```python
from build123d import *

# Parameters (mm, degrees)
CYLINDER014_R     = 1.5
CYLINDER014_DEPTH = 10


with BuildPart() as zylinder014:
    # Cylinder014 → Cylinder014 (new body)
    with BuildSketch(Plane.XY.offset(-17)):
        Circle(CYLINDER014_R)
    extrude(amount=CYLINDER014_DEPTH)


with BuildPart() as cut016:
    # Sketch006 → Revolve001 (revolve)
    with BuildSketch(Plane.XZ):
        Polygon((0, 0), (-3.81, 0), (-5.029301, -1.843205), (-3.199301, -1.843205), (-2.41, -6.74), (-2.41, -14.07), (0, -14.07), align=None)
    revolve(axis=Axis((0, 0, 0), (0, 0, 1)))

    # Cut016: cut Zylinder014
    add(zylinder014.part, mode=Mode.SUBTRACT)


with BuildPart() as cut016_1:
    # Cut016 placement: moved
    add(cut016.part.moved(Location((0, 0, 27.5))))


solid = cut016_1.part
```
The listing builds one solid part. Answer for the finished solid, in the listing's coordinates (mm). A direction names the side the tool comes from. Coordinates: 2 decimals unless noted, no trailing zeros. Write each loop counter-clockwise with the first axis right and the second up, starting at its lowest first coordinate (ties: lowest second). Pieces come first, ordered by that corner, then holes.
Q1. Which of the six approach directions +Z, -Z, +X, -X, +Y, -Y give full straight-line access (tool end or side, diameter ignored) to faces 1 (the flat face through (0, 2, 13.43)), 2 (the flat face through (-1, 3.3, 25.657))?
Returned:
face 1: -Z, +X, -X, +Y, -Y
face 2: -Z
Q2. Section A-A, the plane y = 0 is taken. Write down the section's boundary in (x, z), then the cut area to 3 significant figures.
Returned:
outline: (-5.03, 25.66) - (-3.2, 25.66) - (-2.41, 20.76) - (-2.41, 13.43) - (-1.5, 13.43) - (-1.5, 20.5) - (1.5, 20.5) - (1.5, 13.43) - (2.41, 13.43) - (2.41, 20.76) - (3.2, 25.66) - (5.03, 25.66) - (3.81, 27.5) - (-3.81, 27.5) - close
area: 57.9 mm2
Q3. The mould has two halves that part along Y. Classify faces 3 (the conical face through (-2.586, -0.814, 22.63)), 4 (the flat face through (0, 0, 20.5)), 5 (the flat face through (0, 0, 27.5)): released by +Y, released by -Y, zero draft, split by the parting line, or undercut.
Returned:
face 3: split by the parting line
face 4: undercut
face 5: zero draft
Q4. Given P1, Ø5, axis at x = 0, y = 0, coming from the -Z side; P2, Ø5, axis at x = -3.5, z = 19, coming from the -Y side; P3, Ø1, axis at x = 2, z = 22, coming from the +Y side; P4, Ø3, axis at y = 1.5, z = 18.5, coming from the +X side, each flat-ended and moving along its own axis, determine where each tip first touches the part or whether it passes through.
Returned:
P1: stops at z = 13.43
P2: stops at y = -2.19
P3: stops at y = 2.15
P4: stops at x = 2.41
Q5. Section C-C, the plane z = 19.25 is taken. Write down the section's boundary in (x, y), then the cut area to 3 significant figures.
Returned:
outline: circle Ø4.82 at (0, 0); hole circle Ø3 at (0, 0)
area: 11.2 mm2
Q6. Find the intervals of material crossed by line 1 along Y through (x, z) = (0, 16); line 2 along Y through (x, z) = (1.25, 16.5), in increasing order.
Returned:
line 1: y = -2.41 to -1.5, 1.5 to 2.41
line 2: y = -2.06 to -0.83, 0.83 to 2.06
